```python
from build123d import *

# Parameters (mm, degrees)
F0_W     = 711.2
F0_H     = 609.6
F1_DEPTH = 19.05
F2_W     = 19.05
F2_H     = 577.85
F2_H_2   = 19.05
F2_H_3   = 12.7
F2_W_2   = 673.1
F3_DEPTH = 6.35


with BuildPart() as f1:
    # F0 (on Front) → F1 (new body)
    with BuildSketch(Plane.XZ):
        Rectangle(F0_W, F0_H)
    extrude(amount=F1_DEPTH)

    # F2 (on face) → F3 (cut)
    with BuildSketch(Plane.XZ.offset(19.05)):
        with Locations((-346.075, 15.875)):
            Rectangle(F2_W, F2_H)
        with Locations((-346.075, -282.575)):
            Rectangle(F2_W, F2_H_2)
        with Locations((-346.075, -298.45)):
            Rectangle(F2_W, F2_H_3)
        with Locations((0, -282.575)):
            Rectangle(F2_W_2, F2_H_2)
        with Locations((346.075, -282.575)):
            Rectangle(F2_W, F2_H_2)
        with Locations((346.075, 15.875)):
            Rectangle(F2_W, F2_H)
        with Locations((346.075, -298.45)):
            Rectangle(F2_W, F2_H_3)
    extrude(amount=-F3_DEPTH, mode=Mode.SUBTRACT)


solid = f1.part
```
Geometry: final body of the model. Coordinates: model frame, mm. Round coordinates to 2 decimals unless told otherwise and drop trailing zeros. Order: outer loops, then holes, each group sorted by start corner. A loop starts at its lowest first (then second) coordinate and runs counter-clockwise, first axis right, second up. Notation, with made-up numbers: M -32,85.25 L 11,85.25 A10 cw 11,101.25 Z; hole C 31,9.5 d4. An arc over 180 degrees is marked long. Use one line per item in the form item = value. Start each with the question number.
Q1. Pin query (flat end, axial travel): pin 1 Ø5 at (y, z) = (-15.5, 84.5) entering from +X; pin 2 Ø5 at (y, z) = (-17.5, 113.5) entering from -X. Return the tip coordinate at first contact, or that it passes through.
Q2. Material intervals for line 1 (X direction, y = -15.75, z = 257), sorted ascending. Write a range as [from, to].
Q3. Cut plane A-A (z = 258.5). Return loops of the section in (x, y), and give its area (3 significant figures).
Geometry results:
q1.pin_1 = 336.55
q1.pin_2 = -336.55
q2.line_1 = [-336.55, 336.55]
q3.outline = M -355.6,-12.7 L -336.55,-12.7 L -336.55,-19.05 L 336.55,-19.05 L 336.55,-12.7 L 355.6,-12.7 L 355.6,0 L -355.6,0 Z
q3.area = 13,300 mm^2
